Build history of the part. All positions in model axes, mm. Face numbers are marked on the shaded views. A direction names the side the tool comes from. Round coordinates to 2 decimals unless told otherwise and drop trailing zeros. Write each loop counter-clockwise with the first axis right and the second up, starting at its lowest first coordinate (ties: lowest second). Pieces come first, ordered by that corner, then holes.
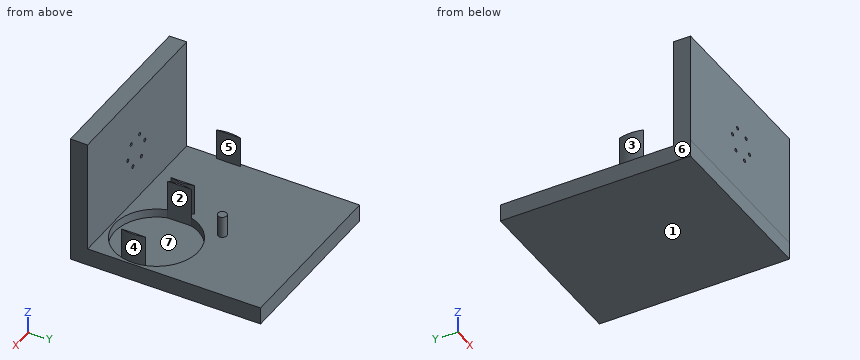
from build123d import *

# Parameters (mm, degrees)
SKETCH_1_W          = 200
SKETCH_1_H          = 200
EXTRUDE_2_DEPTH     = 20
EXTRUDE_5_DEPTH     = 35.7
EXTRUDE_7_DEPTH     = 35.7
SKETCH_16_W         = 200
SKETCH_16_H         = 20
EXTRUDE_9_DEPTH     = 130
SKETCH_17_W         = 20
SKETCH_17_H         = 19.997799489
EXTRUDE_10_DEPTH    = 200
SKETCH_18_R         = 2
CUT_EXTRUDE_3_DEPTH = 20
CUT_EXTRUDE_START   = -10
CUT_EXTRUDE_4_DEPTH = 10
SKETCH_20_R         = 5
EXTRUDE_11_DEPTH    = 25


with BuildPart() as part:
    # Sketch 1 → Extrude 2 (new body)
    with BuildSketch(Plane.XY):
        with Locations((-1.837901133, -0.53181486)):
            Rectangle(SKETCH_1_W, SKETCH_1_H)
    extrude(amount=EXTRUDE_2_DEPTH)

    # Sketch 7 → Extrude 5 (add)
    with BuildSketch(Plane.XY.offset(20)):
        with BuildLine():
            Line((1.147412205, -36.2889375), (1.147412205, -63.78439167))
            ThreePointArc((1.147412205, -63.78439167), (-0.852587795, -50.036664585), (1.147412205, -36.2889375))
        make_face()
        with BuildLine():
            Line((93.647412205, -36.2889375), (93.647412205, -63.78439167))
            ThreePointArc((93.647412205, -63.78439167), (95.647412205, -50.036664585), (93.647412205, -36.2889375))
        make_face()
    extrude(amount=EXTRUDE_5_DEPTH)

    # Sketch 11 → Extrude 7 (add)
    with BuildSketch(Plane.XY.offset(20)):
        with BuildLine():
            Line((-98.401360019, -36.468628425), (-98.401360019, -63.964082595))
            ThreePointArc((-98.401360019, -63.964082595), (-100.401360019, -50.21635551), (-98.401360019, -36.468628425))
        make_face()
        with BuildLine():
            Line((-5.901360019, -36.468628425), (-5.901360019, -63.964082595))
            ThreePointArc((-5.901360019, -63.964082595), (-3.901360019, -50.21635551), (-5.901360019, -36.468628425))
        make_face()
    extrude(amount=EXTRUDE_7_DEPTH)



with BuildPart() as body_2:
    # Sketch 16 → Extrude 9 (new body)
    with BuildSketch(Plane.XY.offset(20)):
        with Locations((-1.837901133, -110.53181486)):
            Rectangle(SKETCH_16_W, SKETCH_16_H)
    extrude(amount=EXTRUDE_9_DEPTH)


with BuildPart() as part_1:
    add(part.part)

    add(body_2.part)  # Extrude 10 merges body 2
    # Sketch 17 → Extrude 10 (add)
    with BuildSketch(Plane(origin=(98.162098867, 0, 0), x_dir=(0, 0, -1), z_dir=(1, 0, 0))):
        with Locations((-10, -110.530714605)):
            Rectangle(SKETCH_17_W, SKETCH_17_H)
    extrude(amount=-EXTRUDE_10_DEPTH)

    # Sketch 18 → Cut-Extrude 3 (cut)
    with BuildSketch(Plane(origin=(0, -100.53181486, 0), x_dir=(1, 0, 0), z_dir=(0, 1, 0))):
        with Locations(Location((-17.139851229, -81.946278464, 0), (0, 0, 270))):
            Circle(SKETCH_18_R)
        with Locations(Location((-10.255452207, -66.129592651, 0), (0, 0, 270))):
            Circle(SKETCH_18_R)
        with Locations(Location((6.884399022, -64.183314187, 0), (0, 0, 270))):
            Circle(SKETCH_18_R)
        with Locations(Location((17.139851229, -78.053721536, 0), (0, 0, 270))):
            Circle(SKETCH_18_R)
        with Locations(Location((10.255452207, -93.870407349, 0), (0, 0, 270))):
            Circle(SKETCH_18_R)
        with Locations(Location((-6.884399022, -95.816685813, 0), (0, 0, 270))):
            Circle(SKETCH_18_R)
    extrude(amount=-CUT_EXTRUDE_3_DEPTH, mode=Mode.SUBTRACT)

    # Sketch 14 → Cut-Extrude 4 (cut)
    with BuildSketch(Plane.XY.offset(20).offset(CUT_EXTRUDE_START)):
        with BuildLine():
            Line((1.147412205, -36.2889375), (1.147412205, -63.78439167))
            ThreePointArc((1.147412205, -63.78439167), (47.397412205, -98.286664585), (93.647412205, -63.78439167))
            Line((93.647412205, -63.78439167), (93.647412205, -36.2889375))
            ThreePointArc((93.647412205, -36.2889375), (47.397412205, -1.786664585), (1.147412205, -36.2889375))
        make_face()
    extrude(amount=CUT_EXTRUDE_4_DEPTH, mode=Mode.SUBTRACT)

    # Sketch 20 → Extrude 11 (add)
    with BuildSketch(Plane.XY.offset(20)):
        with Locations((9.771333485, 4.580206065)):
            Circle(SKETCH_20_R)
    extrude(amount=EXTRUDE_11_DEPTH)


solid = part_1.part
1) Which spindle directions (+Z, -Z, +X, -X, +Y, -Y) get a long thin tool onto all of the face, cutting with end or side? Do the marked faces 4, 5, 6 and 7. Say none if no direction does.
Results:
face 4: +Z, +X
face 5: +Z, +Y
face 6: +Z, -Z, -X, +Y, -Y
face 7: +Z
2) Slice it at D-D (z = 116). Write the cut outline in (x, y).
Results:
outline: (-101.84, -120.53) - (98.16, -120.53) - (98.16, -100.53) - (-101.84, -100.53) - close
3) Mould opens along X. For the marked faces 1, 2 and 3 say: released by +X, released by -X, zero draft, split by the parting line, or undercut.
Results:
face 1: zero draft
face 2: undercut
face 3: released by -X
4) Pin check, flat tips, straight feed: pin 1 Ø4.5 at (x, z) = (-6.88, 95.82) entering from +Y; pin 2 Ø3 at (x, y) = (54, 19) entering from -Z; pin 3 Ø2 at (x, y) = (-48, 74) entering from +Z; pin 4 Ø10 at (x, z) = (13.5, 6) entering from -Y. Stop position of each tip, or through.
Results:
pin 1: stops at y = -100.53
pin 2: stops at z = 0
pin 3: stops at z = 20
pin 4: stops at y = -120.53
5) Slice it at A-A (z = 40). Write the cut outline in (x, y), plus the area to 3 significant figures.
Results:
outline: (-101.84, -120.53) - (98.16, -120.53) - (98.16, -100.53) - (-101.84, -100.53) - close; (-98.4, -63.96) - (-98.4, -36.47) arc R48.25 ccw to start; (-5.9, -63.96) arc R48.25 ccw to (-5.9, -36.47) - close; (1.15, -63.78) - (1.15, -36.29) arc R48.25 ccw to start; circle Ø10 at (9.77, 4.58); (93.65, -63.78) arc R48.25 ccw to (93.65, -36.29) - close
area: 4,230 mm2
6) Slice it at C-C (y = -58). Write the cut outline in (x, z).
Results:
outline: (-101.84, 0) - (98.16, 0) - (98.16, 20) - (94.99, 20) - (94.99, 55.7) - (93.65, 55.7) - (93.65, 10) - (1.15, 10) - (1.15, 55.7) - (-0.19, 55.7) - (-0.19, 20) - (-4.53, 20) - (-4.53, 55.7) - (-5.9, 55.7) - (-5.9, 20) - (-98.4, 20) - (-98.4, 55.7) - (-99.77, 55.7) - (-99.77, 20) - (-101.84, 20) - close
7) Wall check: L1, parallel to Z at x = -40, y = 10.5; L2, parallel to Y at x = 29, z = 77.5; L3, parallel to Z at x = 46, y = -84. Give the ranges that are in metal, low to high.
Results:
L1: z = 0 to 20
L2: y = -120.53 to -100.53
L3: z = 0 to 10
